Autodesk Inventor part; units mm, degrees
ref_plane "Work Plane2" through (25.4, 0, 0) normal (1, 0, 0) x (0, 1, 0)
ref_plane "Work Plane4" through (-25.4, 0, 0) normal (1, 0, 0) x (0, 1, 0)
ref_plane "Work Plane5" through (0, 0, 0) normal (1, 0, 0) x (0, 1, 0)
sketch "Sketch3" plane through (0, 0, 0) normal (0, 0, 1) x (1, 0, 0)
  circle A0 centre (0, 0) radius 25.4
  dimension "d5" = 50.8
ref_plane "Work Plane1" through (12.7, 0, 0) normal (1, 0, 0) x (0, 1, 0)
ref_plane "Work Plane2" through (25.4, 0, 0) normal (1, 0, 0) x (0, 1, 0)
ref_plane "Work Plane4" through (-25.4, 0, 0) normal (1, 0, 0) x (0, 1, 0)
ref_plane "Work Plane3" through (-12.7, 0, 0) normal (1, 0, 0) x (0, 1, 0)
sketch "Sketch4" plane through (25.4, 0, 0) normal (1, 0, 0) x (0, 1, 0)
  line L0 (0, 0) -> (0, 0.0003)
  line L1 (0, 0) -> (0.0003, 0)
  line L2 (0.0003, 0) -> (0, 0.0003)
  dimension "d10" = 0.0003
  dimension "d11" = 0.0003
sketch "Sketch5" plane through (-25.4, 0, 0) normal (1, 0, 0) x (0, 1, 0)
  line L0 (0, 0) -> (0, 0.0003)
  line L1 (0, 0) -> (0.0003, 0)
  line L2 (0.0003, 0) -> (0, 0.0003)
  dimension "d12" = 0.0003
  dimension "d13" = 0.0003
ref_plane "Work Plane5" through (0, 0, 0) normal (1, 0, 0) x (0, 1, 0)
sketch "Sketch6" plane through (-12.7, 0, 0) normal (1, 0, 0) x (0, 1, 0)
  line L0 (0, 0) -> (21.997, 0)
  line L1 (0, 0) -> (-21.997, 0)
  line L2 (-21.997, 0) -> (-21.997, 43.9941)
  line L3 (-21.997, 43.9941) -> (21.997, 0)
  dimension "d15" = 21.9971
  dimension "d16" = 21.9971
  dimension "d17" = 43.9941
sketch "Sketch7" plane through (12.7, 0, 0) normal (1, 0, 0) x (0, 1, 0)
  line L0 (0, 0) -> (21.997, 0)
  line L1 (0, 0) -> (-21.997, 0)
  line L2 (-21.997, 0) -> (-21.997, 43.9941)
  line L3 (-21.997, 43.9941) -> (21.997, 0)
  dimension "d18" = 21.9971
  dimension "d19" = 21.9971
  dimension "d20" = 43.9941
sketch "Sketch8" plane through (0, 0, 0) normal (1, 0, 0) x (0, 1, 0)
  line L0 (0, 0) -> (25.4, 0)
  line L1 (0, 0) -> (-25.4, 0)
  line L2 (-25.4, 0) -> (-25.4, 50.8)
  line L3 (-25.4, 50.8) -> (25.4, 0)
  dimension "d21" = 25.4
  dimension "d22" = 25.4
  dimension "d23" = 50.8
extrude "Extrusion2" add sketch "Sketch8" along normal mid plane 12.7
extrude "Extrusion3" add sketch "Sketch7" along normal mid plane 12.7
extrude "Extrusion4" add sketch "Sketch6" along normal mid plane 12.7
sketch "Sketch9" plane through (19.05, 0, 0) normal (1, 0, 0) x (0, 0, -1)
  line L0 (0, 0) -> (0, 15.24)
  line L1 (0, -21.997) -> (0, 21.997)
  line L2 (0, 0) -> (0, -15.24)
  line L3 (0, -15.24) -> (-30.48, -15.24)
  line L4 (-30.48, -15.24) -> (0, 15.24)
  dimension "d40" = 15.24
  dimension "d41" = 15.24
  dimension "d42" = 30.48
sketch "Sketch10" plane through (-19.05, 0, 0) normal (-1, 0, 0) x (0, 0, 1)
  line L0 (0, 0) -> (0, 15.24)
  line L1 (0, -21.997) -> (0, 21.997)
  line L2 (0, 0) -> (0, -15.24)
  line L3 (0, -15.24) -> (-30.48, -15.24)
  line L4 (-30.48, -15.24) -> (0, 15.24)
  line L5 (0, -15.24) -> (30.48, -15.24)
  line L6 (30.48, -15.24) -> (0, 15.24)
  dimension "d43" = 15.24
  dimension "d44" = 15.24
  dimension "d45" = 30.48
extrude "Extrusion5" add sketch "Sketch10" along normal blind 6.35 contours L0 L6 L5 L1
extrude "Extrusion6" add sketch "Sketch9" along normal blind 6.35
chamfer "Chamfer1" distance 3.175 angle 45 12 edges at (19.05, -21.997, 21.997) (25.4, -15.24, 15.24) (25.4, 0, 15.24) (19.05, 0, 21.997) (6.35, -25.4, 25.4) (6.35, 0, 25.4) (-6.35, 0, 25.4) (-6.35, -25.4, 25.4) (-19.05, 0, 21.997) (-19.05, -21.997, 21.997) (-25.4, 0, 15.24) (-25.4, -15.24, 15.24)
properties part number "crossection_3DPrint"
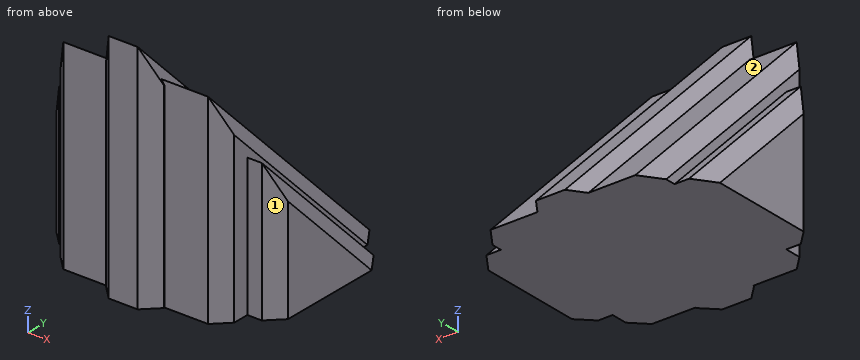
Source: CAD feature listing. Evaluate the final solid. Frame: model axes, mm. Face numbers are marked on the shaded views. A direction names the side the tool comes from. Round coordinates to 2 decimals unless told otherwise and drop trailing zeros. Loops run counter-clockwise (first coordinate to the right, second up) from the corner with the lowest first, then second, coordinate; pieces in that order, holes last. Notation, with made-up numbers: M 80,6.25 L 85,6.25 A9 ccw 85,12.25 Z; hole C 20.25,3 d6. An arc over 180 degrees is marked long. Return JSON: item names as keys, results as strings. Group by question number.
1. Material intervals for line 1 along X through (y, z) = (6, 11.5); line 2 along Z through (x, y) = (-11, -19); line 3 along Z through (x, y) = (-13.5, 3.5), sorted ascending. Write a range as from..to.
2. Section query B-B on z = 26. Output: boundary loops of the cut face in (x, y) (3 decimals), and give its area (3 significant figures).
3. Section query A-A on y = -1. Output: boundary loops of the cut face in (x, z) (3 decimals).
4. Pin query (flat end, axial travel): pin 1 (10 mm diameter, centred on x = -1.5, y = 5, fed in from +Z); pin 2 (3.5 mm diameter, centred on x = 21, z = 9.5, fed in from -Y); pin 3 (3 mm diameter, centred on y = -6.5, z = 25.5, fed in from -X). Return the tip coordinate at first contact, or that it passes through.
5. Section query C-C on x = 13.5. Output: boundary loops of the cut face in (y, z).
6. Reachability of the marked faces 1 and 2 from +Z, -Z, +X, -X, +Y, -Y: full face, straight path, thin tool, end or side. Return the list, or none.
Checks:
{
 "1": {"line 1": "x = -19.05..19.05", "line 2": "z = 0..41", "line 3": "z = 0..18.5"},
 "2": {"outline": "M -24.081,-13.384 L -22.225,-15.24 L -19.05,-15.24 L -19.05,-18.822 L -15.875,-21.997 L -6.35,-21.997 L -6.35,-22.225 L -3.175,-25.4 L 3.175,-25.4 L 6.35,-22.225 L 6.35,-21.997 L 15.875,-21.997 L 19.05,-18.822 L 19.05,-15.24 L 22.225,-15.24 L 24.081,-13.384 L 22.225,-10.76 L 19.05,-10.76 L 19.05,-8.493 L 15.875,-4.003 L 5.581,-4.003 L 3.175,-0.6 L -3.175,-0.6 L -5.581,-4.003 L -15.875,-4.003 L -19.05,-8.493 L -19.05,-10.76 L -22.225,-10.76 Z", "area": "761 mm²"},
 "3": {"outline": "M -25.4,0 L 25.4,0 L 25.4,11.75 L 22.225,16.24 L 19.05,16.24 L 19.05,18.507 L 15.875,22.997 L 5.581,22.997 L 3.175,26.4 L -3.175,26.4 L -5.581,22.997 L -15.875,22.997 L -19.05,18.507 L -19.05,16.24 L -22.225,16.24 L -25.4,11.75 Z"},
 "4": {"pin 1": "stops at z = 25.4", "pin 2": "stops at y = -15.24", "pin 3": "stops at x = -19.05"},
 "5": {"outline": "M -22,0 L 22,0 L -22,43.99 Z"},
 "6": {"face 1": "+Z, -Z, +X, -Y", "face 2": "+Z, -X, +Y"}
}
